```python
from build123d import *

# Parameters (mm, degrees)
F0_R          = 16.8275
F1_DEPTH      = 25.4
F1_DEPTH_BACK = 31.75
F3_R          = 14.605
F4_DEPTH      = 12.7
F6_W          = 26.67
F6_H          = 17.78
F7_DEPTH      = 25.4


with BuildPart() as f1:
    # F0 (on Top) → F1 (new body, two sides)
    with BuildSketch(Plane.XY) as f1_sk:
        Circle(F0_R)
    extrude(amount=F1_DEPTH)
    extrude(f1_sk.sketch, amount=-F1_DEPTH_BACK)

    # F3 (on offset) → F4 (cut)
    with BuildSketch(Plane.XY.offset(25.4)):
        Circle(F3_R)
    extrude(amount=-F4_DEPTH, mode=Mode.SUBTRACT)

    # F6 (on offset) → F7 (cut)
    with BuildSketch(Plane(origin=(0, 0, -31.75), x_dir=(1, 0, 0), z_dir=(0, 0, -1))):
        Rectangle(F6_W, F6_H)
    extrude(amount=-F7_DEPTH, mode=Mode.SUBTRACT)


solid = f1.part
```
Source: CAD feature listing. Evaluate the final solid. Frame: model axes, mm. A direction names the side the tool comes from. Round coordinates to 2 decimals unless told otherwise and drop trailing zeros. Loops run counter-clockwise (first coordinate to the right, second up) from the corner with the lowest first, then second, coordinate; pieces in that order, holes last. Notation, with made-up numbers: M 40.25,-12.75 L 66.25,-12.75 A23 ccw 66.25,16.25 Z; hole C 7.25,36.25 d11. An arc over 180 degrees is marked long. Use a Markdown table: item, result. Add a question column.
1. Set-up query: faces 5 (the flat face through (0, 0, 12.7)), 6 (the flat face through (0, -8.89, -19)), 7 (the flat face through (-5, 14, 25.4)). Return all of +Z, -Z, +X, -X, +Y, -Y with unobstructed straight access to the full face (end or side cutting, diameter ignored); none if empty.
2. Pull-direction query (Y, two-part tool) for faces 1 (the cylindrical face through (-10.764, 9.871, 19.139)), 2 (the flat face through (-13.335, 0, -19)), 3 (the flat face through (0, -11, -31.75)), 4 (the cylindrical face through (-3.648, -16.427, -2.775)); classes: +Y half, -Y half, draft (parallel to the pull), parting line (faces both ways), or undercut.
3. Contact query for flat-ended pins moving along their axis: pin 1 (12 mm diameter, centred on x = -7, z = -4, fed in from +Y); pin 2 (9 mm diameter, centred on x = 3, y = -3.5, fed in from +Z); pin 3 (4 mm diameter, centred on x = -9.5, z = 2.5, fed in from +Y). Output: stop coordinate, or through.
4. Ray query, line 1 along Y through (x, z) = (0, 15.5) (1 decimal); line 2 along X through (y, z) = (-4, -21) (3 decimals); line 3 along Z through (x, y) = (1, 1). Return the intervals inside material, ascending. Write a range as [from, to].
5. Cut plane A-A, the plane z = -8. Output: boundary loops of the cut face in (x, y) (1 decimal).
6. Cut plane D-D, the plane z = 12. Output: boundary loops of the cut face in (x, y) (1 decimal).
Solution:
| question | item | result |
|---|---|---|
| 1 | face 5 | +Z |
| 1 | face 6 | -Z |
| 1 | face 7 | +Z, +X, -X, +Y, -Y |
| 2 | face 1 | undercut |
| 2 | face 2 | undercut |
| 2 | face 3 | draft |
| 2 | face 4 | parting line |
| 3 | pin 1 | stops at y = 16.8 |
| 3 | pin 2 | stops at z = 12.7 |
| 3 | pin 3 | stops at y = 15.06 |
| 4 | line 1 | y = [-16.8, -14.6], [14.6, 16.8] |
| 4 | line 2 | x = [-16.345, -13.335], [13.335, 16.345] |
| 4 | line 3 | z = [-6.35, 12.7] |
| 5 | outline | C 0,0 d33.7; hole M -13.3,-8.9 L 13.3,-8.9 L 13.3,8.9 L -13.3,8.9 Z |
| 6 | outline | C 0,0 d33.7 |
